Geometry check sheet. Reference: drawing and pictorial views, mm from the part's lowest x, y, z. A direction names the side the tool comes from. Give positions to 0.01 mm unless a question says otherwise; leave off trailing zeros. Loops run counter-clockwise (first coordinate to the right, second up) from the corner with the lowest first, then second, coordinate; pieces in that order, holes last. Notation, with made-up numbers: (0, 44.25) -> (25, 44.25) arc R7 cw to (25, 49.25) -> close; hole circle Ø1 at (17, 68). An arc over 180 degrees is marked (long way). Answer in a Markdown table with one row per item. Add a question column.
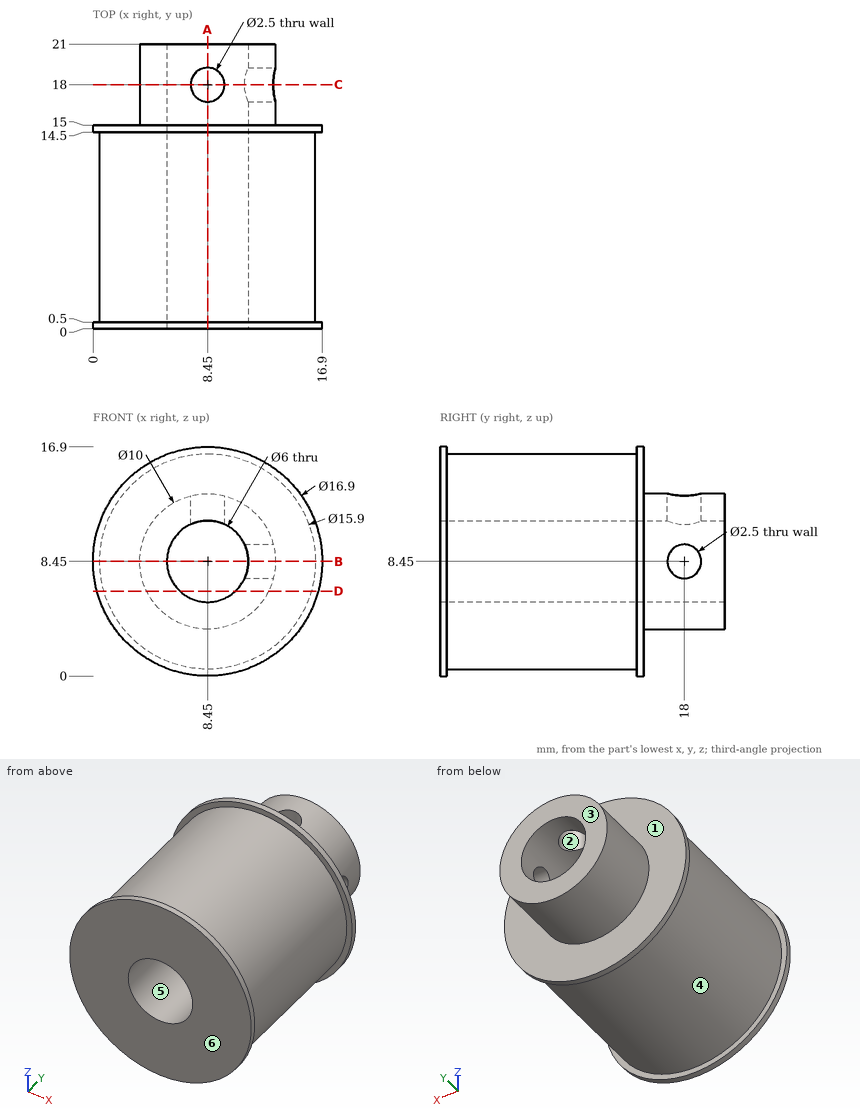
1. Sectioned sample at B-B (z = 8.45). Enter the section's corners in (x, y).
2. Sectioned sample at D-D (z = 6.25). Enter the section's corners in (x, y).
3. Gauge pin test, flat ends, axial feed: pin 1 Ø7 at (x, z) = (8.45, 8.45) entering from +Y; pin 2 Ø2 at (y, z) = (18, 8.45) entering from -X; pin 3 Ø3 at (x, y) = (8.45, 18) entering from -Z; pin 4 Ø3 at (x, y) = (4.5, 3.5) entering from -Z. Record the tip position at first contact, or that the pin passes through.
4. Release check for a two-part mould opening along X. For the marked faces 4, 5 and 6 record: released by +X, released by -X, zero draft, split by the parting line, or undercut.
5. Sectioned sample at C-C (y = 18). Enter the section's corners in (x, z), plus the area to 3 significant figures.
6. Sectioned sample at A-A (x = 8.45). Enter the section's corners in (y, z).
7. Access from +Z, -Z, +X, -X, +Y, -Y to the whole of each face (thin tool, end or side, straight path). Record for the marked faces 1, 2 and 3.
8. Material ranges on L1, parallel to Y at x = 12.05, z = 8.45; L2, parallel to X at y = 16.75, z = 9, recorded low to high. Write a range as from..to.
Response:
| question | item | result |
|---|---|---|
| 1 | outline | (0, 0) -> (5.45, 0) -> (5.45, 21) -> (3.45, 21) -> (3.45, 15) -> (0, 15) -> (0, 14.5) -> (0.5, 14.5) -> (0.5, 0.5) -> (0, 0.5) -> close; (11.45, 0) -> (16.9, 0) -> (16.9, 0.5) -> (16.4, 0.5) -> (16.4, 14.5) -> (16.9, 14.5) -> (16.9, 15) -> (13.45, 15) -> (13.45, 16.75) -> (11.45, 16.75) -> close; (11.45, 19.25) -> (13.45, 19.25) -> (13.45, 21) -> (11.45, 21) -> close |
| 2 | outline | (0.29, 0) -> (6.41, 0) -> (6.41, 21) -> (3.96, 21) -> (3.96, 15) -> (0.29, 15) -> (0.29, 14.5) -> (0.81, 14.5) -> (0.81, 0.5) -> (0.29, 0.5) -> close; (10.49, 0) -> (16.61, 0) -> (16.61, 0.5) -> (16.09, 0.5) -> (16.09, 14.5) -> (16.61, 14.5) -> (16.61, 15) -> (12.94, 15) -> (12.94, 21) -> (10.49, 21) -> close |
| 3 | pin 1 | stops at y = 21 |
| 3 | pin 2 | stops at x = 3.45 |
| 3 | pin 3 | stops at z = 3.45 |
| 3 | pin 4 | stops at z = 0.89 |
| 4 | face 4 | split by the parting line |
| 4 | face 5 | undercut |
| 4 | face 6 | zero draft |
| 5 | outline | (7.2, 11.18) -> (7.2, 13.29) arc R5 ccw (long way) to (13.29, 7.2) -> (11.18, 7.2) arc R3 cw (long way) to start; (9.7, 11.18) arc R3 cw to (11.18, 9.7) -> (13.29, 9.7) arc R5 ccw to (9.7, 13.29) -> close |
| 5 | area | 40.1 mm2 |
| 6 | outline | (0, 0) -> (0.5, 0) -> (0.5, 0.5) -> (14.5, 0.5) -> (14.5, 0) -> (15, 0) -> (15, 3.45) -> (21, 3.45) -> (21, 5.45) -> (0, 5.45) -> close; (0, 11.45) -> (16.75, 11.45) -> (16.75, 13.45) -> (15, 13.45) -> (15, 16.9) -> (14.5, 16.9) -> (14.5, 16.4) -> (0.5, 16.4) -> (0.5, 16.9) -> (0, 16.9) -> close; (19.25, 11.45) -> (21, 11.45) -> (21, 13.45) -> (19.25, 13.45) -> close |
| 7 | face 1 | +Y |
| 7 | face 2 | +Z |
| 7 | face 3 | +Z, -Z, +X, -X, +Y |
| 8 | L1 | y = 0..16.75, 19.25..21 |
| 8 | L2 | x = 3.48..5.5, 11.4..13.42 |
